```python
from build123d import *

# Parameters (mm, degrees)
SKETCH1_W           = 25.4
SKETCH1_H           = 76.2
BOSS_EXTRUDE1_DEPTH = 19.05
SKETCH2_W           = 19.05
SKETCH2_H           = 19.05
CUT_EXTRUDE1_DEPTH  = 50.595085442
CUT_EXTRUDE2_REACH  = 57.358
SKETCH4_R           = 3.96875


with BuildPart() as part:
    # Sketch1 → Boss-Extrude1 (new, symmetric)
    with BuildSketch(Plane.XY):
        Rectangle(SKETCH1_W, SKETCH1_H)
    extrude(amount=BOSS_EXTRUDE1_DEPTH, both=True)

    # Sketch2 → Cut-Extrude1 (cut, through all)
    with BuildSketch(Plane(origin=(12.7, 0, 0), x_dir=(0, 0, -1), z_dir=(1, 0, 0))):
        with Locations((0, 28.575)):
            Rectangle(SKETCH2_W, SKETCH2_H)
    extrude(amount=-CUT_EXTRUDE1_DEPTH, mode=Mode.SUBTRACT)

    # Cut-Extrude2: up to this face of the body (flat: up to its plane)
    cut_extrude2_end = Plane(part.part.faces().sort_by_distance((0, 0, -19.05))[0])
    # Sketch4 → Cut-Extrude2 (cut, up to the picked face)
    with BuildSketch(Plane.XY.offset(19.05), mode=Mode.PRIVATE) as cut_extrude2_sk1:
        with Locations((0, 28.575)):
            Circle(SKETCH4_R)
    cut_extrude2_tool1 = split(extrude(cut_extrude2_sk1.sketch, amount=-CUT_EXTRUDE2_REACH, mode=Mode.PRIVATE), bisect_by=cut_extrude2_end, keep=Keep.BOTH, mode=Mode.PRIVATE)
    add(cut_extrude2_tool1.solids().sort_by(Axis((0, 28.575, 19.05), (0, 0, -1)))[0], mode=Mode.SUBTRACT)


solid = part.part
```
Could you check a few things on this model? Use its own coordinates, in mm. A direction names the side the tool comes from. Coordinates: 2 decimals unless noted, no trailing zeros. Loops run counter-clockwise (first coordinate to the right, second up) from the corner with the lowest first, then second, coordinate; pieces in that order, holes last.
1) Thinking about a two-plate mould opening in Z: for faces 1 (the face through (0, 33, 9.525)), 2 (the face through (0, -38.1, 0)), 3 (the face through (0, 1, 19.05)), which applies, released by +Z, released by -Z, zero draft, split by the parting line, or undercut?
Reported:
face 1: undercut
face 2: zero draft
face 3: released by +Z
2) Imagine slicing it at A-A (x = -8.5). List the corners of the cut face in (y, z) for me (3 decimals).
Reported:
outline: (-38.1, -19.05) - (38.1, -19.05) - (38.1, -9.525) - (19.05, -9.525) - (19.05, 9.525) - (38.1, 9.525) - (38.1, 19.05) - (-38.1, 19.05) - close
3) Please list where these lines run through material, in increasing order: line 1 along Y through (x, z) = (0, 15); line 2 along Y through (x, z) = (-0.75, 14); line 3 along Y through (x, z) = (11.5, -7).
Reported:
line 1: y = -38.1 to 24.61, 32.54 to 38.1
line 2: y = -38.1 to 24.68, 32.47 to 38.1
line 3: y = -38.1 to 19.05
4) Which directions (+Z, -Z, +X, -X, +Y, -Y) give clear straight access to the entire face, cutting with the end or side of a thin tool? Please do faces 4 (the face through (2.134, 31.921, -14.221)), 5 (the face through (0, 33, -9.525)).
Reported:
face 4: +Z, -Z
face 5: +X, -X, +Y
5) Imagine slicing it at C-C (z = -1.5). List the corners of the cut face in (x, y) for me.
Reported:
outline: (-12.7, -38.1) - (12.7, -38.1) - (12.7, 19.05) - (-12.7, 19.05) - close
6) Imagine slicing it at B-B (x = 0). List the corners of the cut face in (y, z) for me (3 decimals), and give its area (3 significant figures).
Reported:
outline: (-38.1, -19.05) - (24.606, -19.05) - (24.606, -9.525) - (19.05, -9.525) - (19.05, 9.525) - (24.606, 9.525) - (24.606, 19.05) - (-38.1, 19.05) - close; (32.544, -19.05) - (38.1, -19.05) - (38.1, -9.525) - (32.544, -9.525) - close; (32.544, 9.525) - (38.1, 9.525) - (38.1, 19.05) - (32.544, 19.05) - close
area: 2,390 mm2
7) Will this pin go through, and if not, where does the flat tip stop? pin 1 Ø12 at (x, z) = (-3, 2) entering from +Y.
Reported:
pin 1: stops at y = 19.05
